Input: part model. Units: mm. Frame: model coordinates. A direction names the side the tool comes from. Round coordinates to 2 decimals unless told otherwise and drop trailing zeros. Loops run counter-clockwise (first coordinate to the right, second up) from the corner with the lowest first, then second, coordinate; pieces in that order, holes last. Notation, with made-up numbers: M -14,-7.5 L -9,-7.5 A30 cw -9,21.5 Z; hole C -22,89 d5. An arc over 180 degrees is marked long. Put each result on its own line as item: value. Start each with the question number.
1) Line query: probe 1 along Z at (x, y) = (37, -16); probe 2 along Y at (x, z) = (61, 3); probe 3 along X at (y, z) = (-14, 36.5). Output: solid intervals per line, ascending.
2) Reachability of faces 4 (the face through (18, -16, 30)), 5 (the face through (0, -16, 8)), 6 (the face through (-24, -19, 13)), 7 (the face through (-5, -16, 64)) from +Z, -Z, +X, -X, +Y, -Y: full face, straight path, thin tool, end or side. Return the list, or none.
3) Draft query along Y for faces 1 (the face through (49, -16, 39)), 2 (the face through (56, -13, 7)), 3 (the face through (40, -16, 64)). Return one class per face: +Y half, -Y half, draft (parallel to the pull), parting line (faces both ways), or undercut.
4) Section C-C on y = -15.5. State how many separate pieces and enclosed holes the cut face has, plus the area to 3 significant figures.
5) Section A-A on z = 54. Output: boundary loops of the cut face in (x, y), plus the area to 3 significant figures.
6) Section B-B on x = -26.5. Output: boundary loops of the cut face in (y, z), plus the area to 3 significant figures.
7) Pin query (flat end, axial travel): pin 1 (7.5 mm diameter, centred on x = -32.5, y = -21.5, fed in from +Z); pin 2 (1 mm diameter, centred on y = -26, z = 19, fed in from +X); pin 3 (16 mm diameter, centred on y = -14, z = 39.5, fed in from -X). Return the tip coordinate at first contact, or that it passes through.
8) Section D-D on z = 46. Output: boundary loops of the cut face in (x, y), plus the area to 3 significant figures.
from build123d import *

# Parameters (mm, degrees)
F1_DEPTH  = 32
F3_DEPTH  = 25
F4_R      = 5.5
F5_DEPTH  = 25
F6_R      = 5.5
F7_DEPTH  = 25
F10_DEPTH = 19
F8_R      = 6.5
F11_DEPTH = 88.001
F13_DEPTH = 19


with BuildPart() as f1:
    # F0 (on Front) → F1 (new body)
    with BuildSketch(Plane.XZ):
        Polygon((-39, 13), (-39, 0), (0, 0), (0, 17), (35, 17), (35, 0), (74, 0), (74, 13), (49, 13), (49, 60.129), (30, 60.129), (30, 30), (5, 30), (5, 60.129), (-14, 60.129), (-14, 13), align=None)
    extrude(amount=F1_DEPTH)

    # F2 (on face) → F3 (cut)
    with BuildSketch(Plane.XY.offset(13)):
        Polygon((-39, -32), (-29, -32), (-39, -22), align=None)
        Polygon((-39, 0), (-39, -10), (-29, 0), align=None)
    extrude(amount=-F3_DEPTH, mode=Mode.SUBTRACT)

    # F4 (on face) → F5 (cut)
    with BuildSketch(Plane.XY.offset(13)):
        with Locations((61.5, -13)):
            Circle(F4_R)
        Polygon((74, -22), (64, -32), (74, -32), align=None)
        Polygon((64, 0), (74, -10), (74, 0), align=None)
    extrude(amount=-F5_DEPTH, mode=Mode.SUBTRACT)

    # F6 (on face) → F7 (cut)
    with BuildSketch(Plane.XY.offset(13)):
        with Locations((-26.5, -13)):
            Circle(F6_R)
    extrude(amount=-F7_DEPTH, mode=Mode.SUBTRACT)

    # F9 (on face) → F10 (join)
    with BuildSketch(Plane.YZ.offset(49)):
        with BuildLine():
            Line((-32, 60.129), (0, 60.129))
            ThreePointArc((0, 60.129), (-16, 64.000235), (-32, 60.129))
        make_face()
    extrude(amount=-F10_DEPTH)

    # F8 (on face) → F11 (cut, through all)
    with BuildSketch(Plane.YZ.offset(49)):
        with Locations((-16, 46)):
            Circle(F8_R)
    extrude(amount=-F11_DEPTH, mode=Mode.SUBTRACT)

    # F12 (on face) → F13 (join)
    with BuildSketch(Plane(origin=(-14, 0, 0), x_dir=(0, -1, 0), z_dir=(-1, 0, 0))):
        with BuildLine():
            Line((0, 60.129), (32, 60.129))
            ThreePointArc((32, 60.129), (16, 64.000235), (0, 60.129))
        make_face()
    extrude(amount=-F13_DEPTH)


solid = f1.part
Geometry results:
1. probe 1: z = 0 to 39.5, 52.5 to 64
1. probe 2: y = -32 to -18.48, -7.52 to 0
1. probe 3: x = -14 to 5, 30 to 49
2. face 4: +Z, +Y, -Y
2. face 5: -Z, +Y, -Y
2. face 6: +Z, -X, +Y, -Y
2. face 7: +Z, +X, -X
3. face 1: draft
3. face 2: undercut
3. face 3: parting line
4. separate pieces: 5
4. enclosed holes: 0
4. area: 2,490 mm²
5. outline: M -14,-32 L 5,-32 L 5,0 L -14,0 Z; M 30,-32 L 49,-32 L 49,0 L 30,0 Z
5. area: 1,220 mm²
6. outline: M -32,0 L -18.5,0 L -18.5,13 L -32,13 Z; M -7.5,0 L 0,0 L 0,13 L -7.5,13 Z
6. area: 273 mm²
7. pin 1: stops at z = 13
7. pin 2: stops at x = 49
7. pin 3: stops at x = -14
8. outline: M -14,-32 L 5,-32 L 5,-22.5 L -14,-22.5 Z; M -14,-9.5 L 5,-9.5 L 5,0 L -14,0 Z; M 30,-32 L 49,-32 L 49,-22.5 L 30,-22.5 Z; M 30,-9.5 L 49,-9.5 L 49,0 L 30,0 Z
8. area: 722 mm²
